Autodesk Inventor part; units mm, degrees
ref_plane "YZ Plane" through (0, 0, 0) normal (1, 0, 0) x (0, 1, 0)
ref_plane "XZ Plane" through (0, 0, 0) normal (0, 1, 0) x (-1, 0, 0)
ref_plane "XY Plane" through (0, 0, 0) normal (0, 0, 1) x (1, 0, 0)
sketch "Sketch1" plane through (0, 0, 0) normal (0, 1, 0) x (-1, 0, 0)
  line L0 (0, 0) -> (-5, 0)
  line L1 (-5, 0) -> (-5, 45)
  line L2 (-5, 45) -> (0, 45)
  line L3 (0, 45) -> (0, 0)
  line L4 (-5, 45) -> (-20, 45)
  line L5 (-20, 45) -> (-20, 40)
  line L6 (-20, 40) -> (-5, 40)
  line L7 (-5, 40) -> (-5, 45)
  line L8 (-5, 0) -> (-20, 0)
  line L9 (-20, 0) -> (-20, 5)
  line L10 (-20, 5) -> (-5, 5)
  line L11 (-5, 5) -> (-5, 0)
  point P0 (-5, 40)
  point P1 (-5, 5)
  dimension "d0" = 5
  dimension "d1" = 5
  dimension "d2" = 5
  dimension "d3" = 15
  dimension "d4" = 15
  dimension "d5" = 35
extrude "Extrusion1" add sketch "Sketch1" along normal blind 20
sketch "Sketch2" plane through (0, 0, 45) normal (0, 0, 1) x (1, 0, 0)
  circle A0 centre (10, 10) radius 2.5
  line L0 (20, 0) -> (20, 20)
  line L1 (20, 0) -> (10, 0)
  line L2 (10, 0) -> (10, 20)
  line L3 (10, 20) -> (20, 20)
  line L4 (20, 20) -> (20, 0)
  line L5 (0, 0) -> (20, 0)
  dimension "d8" = 10
  dimension "d9" = 10
  dimension "d10" = 10
  dimension "d11" = 5
extrude "Extrusion2" cut sketch "Sketch2" against normal blind 200
sketch "Sketch3" plane through (0, 0, 0) normal (-1, 0, 0) x (0, 0, 1)
  line L0 (5, 0) -> (5, 20)
  line L1 (40, 0) -> (40, 20)
  line L2 (5, 15) -> (40, 15)
  line L3 (40, 15) -> (40, 5)
  line L4 (40, 5) -> (5, 5)
  line L5 (5, 5) -> (5, 15)
  line L6 (0, 20) -> (45, 20)
  line L7 (0, 0) -> (45, 0)
  point P0 (5, 5)
  dimension "d14" = 5
  dimension "d15" = 5
extrude "Extrusion3" cut sketch "Sketch3" against normal blind 20 contours L0 L2 L1 L4
sketch "Sketch4" plane through (0, 0, 0) normal (-1, 0, 0) x (0, 0, 1)
  line L0 (45, 0) -> (45, 20)
  line L1 (45, 20) -> (55, 20)
  line L2 (55, 20) -> (55, 0)
  line L3 (55, 0) -> (45, 0)
  line L4 (45, 0) -> (45, 20)
  line L5 (0, 20) -> (0, 12.5)
  line L6 (0, 20) -> (-10, 20)
  line L7 (-10, 20) -> (-10, 0)
  line L8 (-10, 0) -> (0, 0)
  line L9 (0, 0) -> (0, 20)
  circle A0 centre (50, 3) radius 1.375
  circle A1 centre (50, 17) radius 1.375
  circle A2 centre (-5, 17) radius 1.375
  circle A3 centre (-5, 3) radius 1.375
  point P0 (0, 0)
  point P1 (50, 20)
  point P2 (0, 12.5)
  dimension "d18" = 10
  dimension "d19" = 10
  dimension "d20" = 3
  dimension "d21" = 3
  dimension "d22" = 5
  dimension "d23" = 5
  dimension "d24" = 5
  dimension "d25" = 5
  dimension "d26" = 3
  dimension "d27" = 3
  dimension "d28" = 2.75
  dimension "d29" = 2.75
  dimension "d30" = 2.75
  dimension "d31" = 2.75
extrude "Extrusion4" add sketch "Sketch4" against normal blind 5
sketch "Sketch5" plane through (10, 12.5, 45) normal (1, 0, 0) x (0, 0, -1)
  circle A0 centre (42.5, 5) radius 1.375
  circle A1 centre (42.5, -10) radius 1.375
  circle A2 centre (2.5, 5) radius 1.375
  circle A3 centre (2.5, -10) radius 1.375
  line L0 (40, 7.5) -> (45, 7.5)
  line L1 (45, 7.5) -> (45, 0)
  line L2 (45, -5) -> (45, -12.5)
  line L3 (45, -12.5) -> (40, -12.5)
  line L4 (5, -12.5) -> (0, -12.5)
  line L5 (0, -12.5) -> (0, -5)
  line L6 (0, 0) -> (0, 7.5)
  line L7 (0, 7.5) -> (5, 7.5)
  dimension "d34" = 2.5
  dimension "d35" = 2.5
  dimension "d36" = 2.5
  dimension "d37" = 2.5
  dimension "d38" = 2.5
  dimension "d39" = 2.5
  dimension "d40" = 2.5
  dimension "d41" = 2.5
  dimension "d42" = 2.75
  dimension "d43" = 2.75
  dimension "d44" = 2.75
  dimension "d45" = 2.75
extrude "Extrusion5" cut sketch "Sketch5" against normal blind 15
sketch "Sketch6" plane through (0, 0, 55) normal (-1, 0, 0) x (0, 0, 1)
  circle A0 centre (-12.5, 17.5) radius 1.375
  circle A1 centre (-12.5, 17.5) radius 2
  circle A2 centre (-12.5, 2.5) radius 1.375
  circle A3 centre (-12.5, 2.5) radius 2
  circle A4 centre (-52.5, 2.5) radius 1.375
  circle A5 centre (-52.5, 2.5) radius 2
  circle A6 centre (-52.5, 17.5) radius 1.375
  circle A7 centre (-52.5, 17.5) radius 2
  point P0 (-55, 0)
  dimension "d48" = 4
  dimension "d49" = 4
  dimension "d50" = 4
  dimension "d51" = 4
extrude "Extrusion6" cut sketch "Sketch6" against normal blind 5 contours A0 | A1 | A2 | A3 | A4 | A5 | A6 | A7
equation "\"d14\" = d15"
equation "\"d19\" = d18"
equation "\"d20\" = d21"
equation "\"d24\" = d23"
equation "\"d25\" = d22"
equation "\"d26\" = d20"
equation "\"d27\" = d21"
equation "\"d34\" = d35"
equation "\"d37\" = d34"
equation "\"d38\" = d34"
equation "\"d39\" = d36"
equation "\"d40\" = d39"
equation "\"d41\" = d34"
equation "\"d44\" = d42"
equation "\"d45\" = d43"
equation "\"d49\" = d48"
equation "\"d50\" = d49"
equation "\"d51\" = d48"
properties part number "MotorDifferentialMountingBracket"
Design review of the part built by this model. Coordinates are the model's own, in mm. A direction names the side the tool comes from. Round coordinates to 2 decimals unless told otherwise and drop trailing zeros. Loops run counter-clockwise (first coordinate to the right, second up) from the corner with the lowest first, then second, coordinate; pieces in that order, holes last. Notation, with made-up numbers: (0, -5.5) -> (23, -5.5) arc R14 ccw to (23, 12.5) -> close; hole circle Ø3 at (-7.75, 85.5). An arc over 180 degrees is marked (long way). Use one line per item in the form item = value. Start each with the question number.
Q1. Wall thickness on line 1 along Y through (x, z) = (1.85, 42.5); line 2 along Y through (x, z) = (0.75, 5.5); line 3 along Z through (x, y) = (4.75, 5.5): over which ranges is each line inside the solid? List them lowest first. Write a range as [from, to].
Q2. We need section A-A on x = 6. Give the boundary of the cut face in (y, z) (3 decimals), then the cut area to 3 significant figures.
Q3. Machinability: for faces 1 (the face through (5, 18, 4)), 2 (the face through (2, 15, 22)), 3 (the face through (5, 10, 40)), which of the approach directions +Z, -Z, +X, -X, +Y, -Y give a long, thin tool a straight path to every point of the face, cutting with its end or side? Answer none if there is none.
Q4. We need section B-B on y = 11.5. Give the boundary of the cut face in (x, z), then the cut area to 3 significant figures.
Q5. Draft analysis for pull direction Z (two halves, no side actions). For faces 4 (the face through (7.5, 10.1, 42.5)), 5 (the face through (2.465, 2.588, 40.502)), 6 (the face through (7, 10, 45)), state which applies: +Z half, -Z half, draft (parallel to the pull), parting line (faces both ways), or undercut.
Q6. For pin 1 Ø3 at (y, z) = (17, 50) entering from +X; pin 2 Ø5.5 at (x, y) = (8.5, 5.5) entering from -Z; pin 3 Ø1.5 at (x, y) = (8, 7) entering from +Z; pin 4 Ø2.5 at (y, z) = (3, -5) entering from -X, all flat-tipped, find the tip position at first contact; note any pin that passes through.
Q7. We need section D-D on z = 6.5. Give the boundary of the cut face in (x, y), then the cut area to 3 significant figures.
Q8. We need section C-C on z = -5. Give the boundary of the cut face in (x, y) (3 decimals).
Calculated:
q1.line_1 = [0, 0.5], [4.5, 15.5], [19.5, 20]
q1.line_2 = [0, 5], [15, 20]
q1.line_3 = [-10, 5], [40, 55]
q2.outline = (0, 0) -> (20, 0) -> (20, 5) -> (0, 5) -> close; (0, 40) -> (20, 40) -> (20, 45) -> (0, 45) -> close; hole circle Ø2.75 at (2.5, 2.5); hole circle Ø2.75 at (2.5, 42.5); hole circle Ø2.75 at (17.5, 2.5); hole circle Ø2.75 at (17.5, 42.5)
q2.area = 176 mm²
q3.face_1 = -X
q3.face_2 = +X, -X
q3.face_3 = +X
q4.outline = (0, -10) -> (5, -10) -> (5, 0) -> (8, 0) -> (8, 5) -> (0, 5) -> close; (0, 40) -> (8, 40) -> (8, 45) -> (5, 45) -> (5, 55) -> (0, 55) -> close
q4.area = 180 mm²
q5.face_4 = draft
q5.face_5 = undercut
q5.face_6 = +Z half
q6.pin_1 = 5
q6.pin_2 = 0
q6.pin_3 = 45
q6.pin_4 = through
q7.outline = (0, 0) -> (5, 0) -> (5, 5) -> (0, 5) -> close; (0, 15) -> (5, 15) -> (5, 20) -> (0, 20) -> close
q7.area = 50.0 mm²
q8.outline = (0, 0) -> (5, 0) -> (5, 1.625) -> (0, 1.625) -> close; (0, 4.375) -> (5, 4.375) -> (5, 15.625) -> (0, 15.625) -> close; (0, 18.375) -> (5, 18.375) -> (5, 20) -> (0, 20) -> close
